from build123d import *

# Parameters (mm, degrees)
F1_DEPTH   = 30
F2_W       = 3
F2_H       = 25
F1_FACE1_W = 105
F1_FACE1_H = 60
F3_DEPTH   = 14.001
F5_D       = 3.3
F6_R       = 3


with BuildPart() as f1:
    # F0 (on Top) → F1 (new body, symmetric)
    with BuildSketch(Plane.XY):
        with BuildLine():
            Line((-52.5, 0), (52.5, 0))
            ThreePointArc((52.5, 0), (53.2071067812, -0.2928932188), (53.5, -1))
            Line((53.5, -1), (53.5, -12))
            Line((53.5, -12), (55.5, -12))
            Line((55.5, -12), (55.5, -1))
            ThreePointArc((55.5, -1), (54.6213203436, 1.1213203436), (52.5, 2))
            Line((52.5, 2), (-52.5, 2))
            ThreePointArc((-52.5, 2), (-54.6213203436, 1.1213203436), (-55.5, -1))
            Line((-55.5, -1), (-55.5, -12))
            Line((-55.5, -12), (-53.5, -12))
            Line((-53.5, -12), (-53.5, -1))
            ThreePointArc((-53.5, -1), (-53.2071067812, -0.2928932188), (-52.5, 0))
        make_face()
    extrude(amount=F1_DEPTH, both=True)

    # F2 (on face) + F1_face1 (on face) → F3 (cut, through all)
    with BuildSketch(Plane(origin=(0, 2, 0), x_dir=(-1, 0, 0), z_dir=(0, 1, 0))):
        with Locations((-54, 0)):
            Rectangle(F2_W, F2_H)
        with Locations((54, 0)):
            Rectangle(F2_W, F2_H)
    with BuildSketch(Plane.XZ):
        Rectangle(F1_FACE1_W, F1_FACE1_H)
    extrude(amount=-F3_DEPTH, dir=(0, 1, 0), mode=Mode.SUBTRACT)

    # F5 (through all)
    with Locations(Plane.YZ.offset(55.5)):
        with Locations((-6.5, 21.25), (-6.5, -21.25)):
            Hole(F5_D / 2)

    # F6
    f6_edges = [f1.edges().sort_by_distance(p)[0] for p in [
        (-54.5, -12, 30),
        (-54.5, -12, 12.5),
        (-54.5, -12, -12.5),
        (-54.5, -12, -30),
        (54.5, -12, 30),
        (54.5, -12, 12.5),
        (54.5, -12, -12.5),
        (54.5, -12, -30),
    ]]
    fillet(f6_edges, radius=F6_R)


solid = f1.part
Check sheet for the modelled part. Datum: model origin and axes. Units: mm. A direction names the side the tool comes from. Coordinates: 2 decimals unless noted, no trailing zeros. Write each loop counter-clockwise with the first axis right and the second up, starting at its lowest first coordinate (ties: lowest second). Pieces come first, ordered by that corner, then holes. Notation, with made-up numbers: M -28.5,86 L -7.5,86 A21 cw -7.5,108 Z; hole C 14,81 d3. An arc over 180 degrees is marked long. Answer as CSV lines item,"result".
Q1. Go/stop test with flat-tipped pins: pin 1 (1.5 mm diameter, centred on x = 14, z = 10.5, fed in from -Y); pin 2 (1.6 mm diameter, centred on y = 1, z = 2, fed in from +X); pin 3 (0.6 mm diameter, centred on y = 1.5, z = -1.5, fed in from -X). Record where each tip stops, or that it passes through.
Check result:
pin 1,"y = 0"
pin 2,"x = 52.5"
pin 3,"x = -52.5"
Q2. Material ranges on probe 1 along Z at (x, y) = (-54.9, -6.5); probe 2 along X at (y, z) = (-1.5, -15); probe 3 along Y at (x, z) = (30.5, 19), recorded low to high. Write a range as from..to.
Check result:
probe 1,"-30..-22.9, -19.6..-12.5, 12.5..19.6, 22.9..30"
probe 2,"-55.5..-53.5, 53.5..55.5"
probe 3,"0..2"
Q3. Mould release check, pull along Z, two halves, no side actions. Record for faces 1 (the face through (-8, 1, -30)), 2 (the face through (54, -12, 21)), 3 (the face through (54.486, -6.285, -19.614)), 4 (the face through (-54, -3, -12.5)): released by +Z, released by -Z, zero draft, split by the parting line, or undercut.
Check result:
face 1,"released by -Z"
face 2,"zero draft"
face 3,"undercut"
face 4,"undercut"
Q4. Cross-section at C-C (x = -10). Record the boundary of the cut face in (y, z).
Check result:
outline,"M 0,-30 L 2,-30 L 2,30 L 0,30 Z"
Q5. Cross-section at D-D (z = -6.5). Record the boundary of the cut face in (x, y).
Check result:
outline,"M -52.5,0 L 52.5,0 L 52.5,2 L -52.5,2 Z"
Q6. Cross-section at A-A (z = -21.25). Record the boundary of the cut face in (x, y).
Check result:
outline,"M -55.5,-12 L -53.5,-12 L -53.5,-8.15 L -55.5,-8.15 Z; M -55.5,-4.85 L -53.5,-4.85 L -53.5,-1 A1 cw -52.5,0 L 52.5,0 A1 cw 53.5,-1 L 53.5,-4.85 L 55.5,-4.85 L 55.5,-1 A3 ccw 52.5,2 L -52.5,2 A3 ccw -55.5,-1 Z; M 53.5,-12 L 55.5,-12 L 55.5,-8.15 L 53.5,-8.15 Z"
Q7. Set-up check for faces 5 (the face through (-53.5, -7, -23)), 6 (the face through (54.51, -11.1, 13.36)), 7 (the face through (52.5, 1, 0)): record each of +Z, -Z, +X, -X, +Y, -Y from which the full face is reachable in a straight line by a thin tool's end or side.
Check result:
face 5,"+Z, -Z, -Y"
face 6,"+X, -X, -Y"
face 7,"+X, +Y, -Y"
Q8. Cross-section at B-B (y = -7). Count the separate pieces of the cut face and the enclosed holes in it, then the cut area to 3 significant figures.
Check result:
separate pieces,"8"
enclosed holes,"0"
area,"115 mm^2"
